Source: three-view drawing plus pictorial views. Frame: mm from the lowest corner of the part. A direction names the side the tool comes from. Coordinates: 2 decimals unless noted, no trailing zeros. Loops run counter-clockwise (first coordinate to the right, second up) from the corner with the lowest first, then second, coordinate; pieces in that order, holes last. Notation, with made-up numbers: M -19.5,9.5 L 10.5,9.5 A17 cw 10.5,15.5 Z; hole C 79,45 d7. An arc over 180 degrees is marked long. Write each question's results on one line, items separated by ' | '. Start each with the question number.
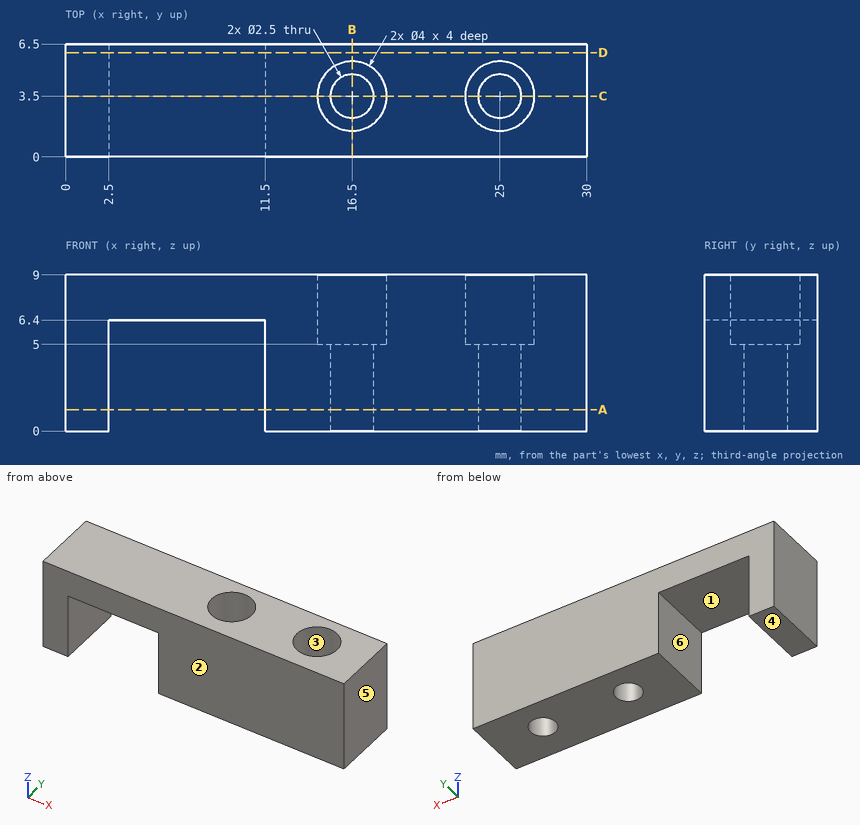
Item 1: Section A-A, the plane z = 1.25. Return loops of the section in (x, y).
Item 2: Pull-direction query (X, two-part tool) for the marked faces 4, 5 and 6; classes: released by +X, released by -X, zero draft, split by the parting line, or undercut.
Item 3: Set-up query: the marked faces 1, 2 and 3. Return all of +Z, -Z, +X, -X, +Y, -Y with unobstructed straight access to the full face (end or side cutting, diameter ignored); none if empty.
Item 4: Section C-C, the plane y = 3.5. Return loops of the section in (x, z).
Item 5: Section B-B, the plane x = 16.5. Return loops of the section in (y, z), plus the area to 3 significant figures.
Item 6: Ray query, L1, parallel to X at y = 3.5, z = 7.2; L2, parallel to X at y = 2.75, z = 8; L3, parallel to X at y = 6, z = 5. Return the intervals inside material, ascending. Write a range as [from, to].
Item 7: Contact query for flat-ended pins moving along their axis: P1, Ø1.2, axis at x = 17, y = 2.5, coming from the +Z side; P2, Ø2, axis at x = 16.5, y = 3.5, coming from the -Z side. Output: stop coordinate, or through.
Item 8: Section D-D, the plane y = 6. Return loops of the section in (x, z), plus the area to 3 significant figures.
Solutions:
1) outline: M 0,0 L 2.5,0 L 2.5,6.5 L 0,6.5 Z; M 11.5,0 L 30,0 L 30,6.5 L 11.5,6.5 Z; hole C 16.5,3.5 d2.5; hole C 25,3.5 d2.5
2) face 4: zero draft | face 5: released by +X | face 6: undercut
3) face 1: -Z, +Y, -Y | face 2: +Z, -Z, +X, -X, -Y | face 3: +Z
4) outline: M 0,0 L 2.5,0 L 2.5,6.4 L 11.5,6.4 L 11.5,0 L 15.25,0 L 15.25,5 L 14.5,5 L 14.5,9 L 0,9 Z; M 17.75,0 L 23.75,0 L 23.75,5 L 23,5 L 23,9 L 18.5,9 L 18.5,5 L 17.75,5 Z; M 26.25,0 L 30,0 L 30,9 L 27,9 L 27,5 L 26.25,5 Z
5) outline: M 0,0 L 2.25,0 L 2.25,5 L 1.5,5 L 1.5,9 L 0,9 Z; M 4.75,0 L 6.5,0 L 6.5,9 L 5.5,9 L 5.5,5 L 4.75,5 Z | area: 30.0 mm²
6) L1: x = [0, 14.5], [18.5, 23], [27, 30] | L2: x = [0, 14.65], [18.35, 23.15], [26.85, 30] | L3: x = [0, 2.5], [11.5, 30]
7) P1: stops at z = 5 | P2: passes through
8) outline: M 0,0 L 2.5,0 L 2.5,6.4 L 11.5,6.4 L 11.5,0 L 30,0 L 30,9 L 0,9 Z | area: 212 mm²
